Build history of the part. All positions in model axes, mm. Face numbers are marked on the shaded views. Give positions to 0.01 mm unless a question says otherwise; leave off trailing zeros. Order: outer loops, then holes, each group sorted by start corner. A loop starts at its lowest first (then second) coordinate and runs counter-clockwise, first axis right, second up. Notation, with made-up numbers: (87, 20.5) - (144, 20.5) arc R28 ccw to (144, 54.5) - close; hole circle Ø1 at (43.5, 19). An arc over 180 degrees is marked (long way). Write each question's results on one line, items separated by ' | '. Start each with the question number.
from build123d import *

# Parameters (mm, degrees)
BOSS_EXTRUDE1_DEPTH     = 2.25
BOSS_EXTRUDE2_DEPTH     = 1.5
CUT_EXTRUDE1_DEPTH      = 4.75
CUT_EXTRUDE1_DEPTH_BACK = 4.75
BOSS_EXTRUDE3_START     = 44.5
SKETCH5_W               = 8
SKETCH5_H               = 12.8
BOSS_EXTRUDE3_DEPTH     = 1.5
BOSS_EXTRUDE4_START     = -44.5
SKETCH5_2_W             = 8
SKETCH5_2_H             = 12.8
BOSS_EXTRUDE4_DEPTH     = 1.5
SKETCH6_R               = 1.2
CUT_EXTRUDE3_DEPTH      = 45.5
CUT_EXTRUDE3_DEPTH_BACK = 45.5
FILLET1_R               = 1.5
FILLET2_R               = 1.5


with BuildPart() as part:
    # Sketch1 → Boss-Extrude1 (new body, symmetric)
    with BuildSketch(Plane(origin=(0, 0, 0), x_dir=(1, 0, 0), z_dir=(0, 1, 0))):
        Polygon((-25.5, -35.5), (25.5, -35.5), (35.5, -31.5), (35.5, 31.5), (25.5, 35.5), (-25.5, 35.5), (-35.5, 31.5), (-35.5, -31.5), align=None)
    extrude(amount=BOSS_EXTRUDE1_DEPTH, both=True)

    # Sketch2 → Boss-Extrude2 (add)
    with BuildSketch(Plane(origin=(0, 2.25, 0), x_dir=(1, 0, 0), z_dir=(0, 1, 0))):
        Polygon((27.233241632, -44.5), (44.5, -37.593296653), (44.5, 37.593296653), (27.233241632, 44.5), (-27.233241632, 44.5), (-44.5, 37.593296653), (-44.5, -37.593296653), (-27.233241632, -44.5), align=None)
    boss_extrude2 = extrude(amount=BOSS_EXTRUDE2_DEPTH)

    # Mirror1: Boss-Extrude2 across plane
    add(boss_extrude2.mirror(Plane.ZX))

    # Sketch3 → Cut-Extrude1 (cut, two sides)
    with BuildSketch(Plane(origin=(0, 0, 0), x_dir=(1, 0, 0), z_dir=(0, 1, 0))) as cut_extrude1_sk:
        Polygon((-25.211126395, -34), (25.211126395, -34), (34, -30.484450558), (34, 30.484450558), (25.211126395, 34), (-25.211126395, 34), (-34, 30.484450558), (-34, -30.484450558), align=None)
    extrude(amount=CUT_EXTRUDE1_DEPTH, mode=Mode.SUBTRACT)
    extrude(cut_extrude1_sk.sketch, amount=-CUT_EXTRUDE1_DEPTH_BACK, mode=Mode.SUBTRACT)

    # Sketch5 → Boss-Extrude3 (add)
    with BuildSketch(Plane.XY.offset(BOSS_EXTRUDE3_START)):
        with Locations((-22, 10.15)):
            Rectangle(SKETCH5_W, SKETCH5_H)
        with Locations((22, 10.15)):
            Rectangle(SKETCH5_W, SKETCH5_H)
    extrude(amount=-BOSS_EXTRUDE3_DEPTH)

    # Sketch5<2> → Boss-Extrude4 (add)
    with BuildSketch(Plane.XY.offset(BOSS_EXTRUDE4_START)):
        with Locations((-22, 10.15)):
            Rectangle(SKETCH5_2_W, SKETCH5_2_H)
        with Locations((22, 10.15)):
            Rectangle(SKETCH5_2_W, SKETCH5_2_H)
    extrude(amount=BOSS_EXTRUDE4_DEPTH)

    # Sketch6 → Cut-Extrude3 (cut, two sides)
    with BuildSketch(Plane.XY) as cut_extrude3_sk:
        with Locations((-22, 13.85)):
            Circle(SKETCH6_R)
        with Locations((22, 13.85)):
            Circle(SKETCH6_R)
        with Locations((-22, 8.45)):
            Circle(SKETCH6_R)
        with Locations((22, 8.45)):
            Circle(SKETCH6_R)
    extrude(amount=CUT_EXTRUDE3_DEPTH, mode=Mode.SUBTRACT)
    extrude(cut_extrude3_sk.sketch, amount=-CUT_EXTRUDE3_DEPTH_BACK, mode=Mode.SUBTRACT)

    # Fillet1
    fillet1_edges = [part.edges().sort_by_distance(p)[0] for p in [
        (35.5, 0, 31.5),
        (25.5, 0, 35.5),
        (0, 2.25, -35.5),
        (0, -2.25, -35.5),
        (35.5, 2.25, 0),
        (35.5, -2.25, 0),
        (-35.5, 2.25, 0),
        (-35.5, -2.25, 0),
        (0, 2.25, 35.5),
        (0, -2.25, 35.5),
        (-25.5, 0, -35.5),
        (-30.5, 2.25, -33.5),
        (-35.5, 0, -31.5),
        (-30.5, -2.25, -33.5),
        (35.5, 0, -31.5),
        (30.5, 2.25, -33.5),
        (25.5, 0, -35.5),
        (30.5, -2.25, -33.5),
        (30.5, 2.25, 33.5),
        (30.5, -2.25, 33.5),
        (-35.5, 0, 31.5),
        (-30.5, 2.25, 33.5),
        (-25.5, 0, 35.5),
        (-30.5, -2.25, 33.5),
        (-22, 3.75, -43),
        (22, 3.75, -43),
        (-22, 3.75, 43),
        (22, 3.75, 43),
        (26, 3.75, 43.75),
        (-18, 3.75, 43.75),
        (18, 3.75, 43.75),
        (-26, 3.75, 43.75),
        (18, 3.75, -43.75),
        (26, 3.75, -43.75),
        (-26, 3.75, -43.75),
    ]]
    fillet(fillet1_edges, radius=FILLET1_R)

    # Fillet2
    fillet2_edges = [part.edges().sort_by_distance(p)[0] for p in [
        (-25.211126395, 0, 34),
        (-34, 0, 30.484450558),
        (-34, 0, -30.484450558),
        (-25.211126395, 0, -34),
        (25.211126395, 0, -34),
        (34, 0, -30.484450558),
        (34, 0, 30.484450558),
        (25.211126395, 0, 34),
    ]]
    fillet(fillet2_edges, radius=FILLET2_R)


solid = part.part
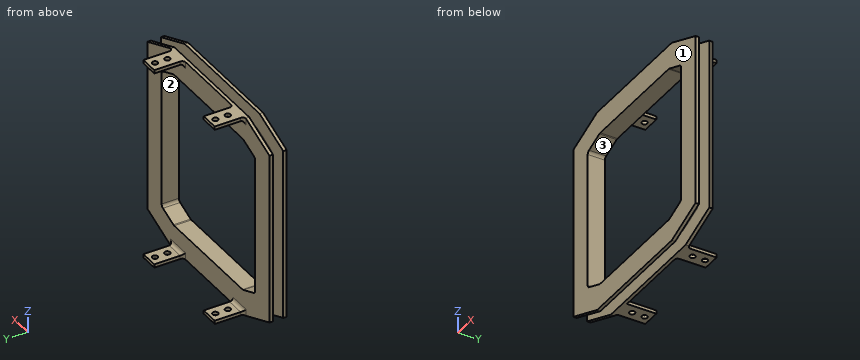
Item 1: Two-plate mould, pull along Z, no slides. Class the marked faces 1, 2 and 3: +Z half, -Z half, draft (parallel to the pull), parting line (faces both ways), or undercut.
Item 2: Flat gauge pins, fed straight in: pin 1 Ø1.7 at (x, y) = (-1, 0) entering from +Z; pin 2 Ø0.8 at (y, z) = (10.5, 43.5) entering from +X; pin 3 Ø1.7 at (y, z) = (0.5, 1.5) entering from +X. Where does each tip first touch, or does it go through?
Item 3: Cut at B-B, the plane y = 13.85. Count the separate pieces of the cut face and the enclosed holes in it, then the cut area to 3 significant figures.
Item 4: Cut at C-C, the plane x = -39. List the corners of the cut face in (y, z), then the cut area to 3 significant figures.
Item 5: Probe line 1 along X through (y, z) = (13.85, 44.1); line 2 along X through (y, z) = (-0.25, 9.5); line 3 along Y through (x, z) = (-37, -35.5). List the from-to ranges inside material, lowest first. Write a range as from..to.
Item 6: Cut at A-A, the plane z = -15.5. List the corners of the cut face in (x, y), then the cut area to 3 significant figures.
Values found:
1) face 1: draft | face 2: undercut | face 3: undercut
2) pin 1: stops at z = 35.5 | pin 2: stops at x = 26 | pin 3: stops at x = 35.63
3) separate pieces: 8 | enclosed holes: 0 | area: 33.6 mm2
4) outline: (-3.75, -39.79) - (-2.25, -39.79) - (-2.25, 39.79) - (-3.75, 39.79) - close; (2.25, -39.79) - (3.75, -39.79) - (3.75, 39.79) - (2.25, 39.79) - close | area: 239 mm2
5) line 1: x = -26..-23.2, -20.8..-18, 18..20.8, 23.2..26 | line 2: x = -35.5..-34, 34..35.5 | line 3: y = -3.75..-2.25, 2.25..3.75
6) outline: (-44.5, -3.75) - (-34, -3.75) - (-34, 3.75) - (-44.5, 3.75) - (-44.5, 2.25) - (-37, 2.25) arc R1.5 cw to (-35.5, 0.75) - (-35.5, -0.75) arc R1.5 cw to (-37, -2.25) - (-44.5, -2.25) - close; (34, -3.75) - (44.5, -3.75) - (44.5, -2.25) - (37, -2.25) arc R1.5 cw to (35.5, -0.75) - (35.5, 0.75) arc R1.5 cw to (37, 2.25) - (44.5, 2.25) - (44.5, 3.75) - (34, 3.75) - close | area: 78.4 mm2
